Geometry check sheet. Reference: the model listing, model coordinates, mm. Face numbers are marked on the shaded views. A direction names the side the tool comes from. Coordinates: 2 decimals unless noted, no trailing zeros. Write each loop counter-clockwise with the first axis right and the second up, starting at its lowest first coordinate (ties: lowest second). Pieces come first, ordered by that corner, then holes. Notation, with made-up numbers: (78.5, 32) -> (109.5, 32) arc R13 ccw to (109.5, 50) -> close; hole circle Ø3 at (42, 12.25). An arc over 180 degrees is marked (long way). Answer in a Markdown table with one row per item. Add a question column.
Q1. Tool access check on the marked faces 4 and 5. Record the directions out of +Z, -Z, +X, -X, +Y, -Y that give a thin tool (end or side, any length) a straight path to the whole face; none if there is none.
Q2. Gauge pin test, flat ends, axial feed: P1, Ø5, axis at y = -19.5, z = 38, coming from the +X side; P2, Ø5.5, axis at x = -3.65, z = 100.03, coming from the -Y side; P3, Ø10, axis at x = 15, z = 12.5, coming from the -Y side; P4, Ø4, axis at y = -18.5, z = 45.5, coming from the +X side. Record the tip position at first contact, or that the pin passes through.
Q3. Section check A-A, the plane y = -11.5. Count the separate pieces of the cut face and the enclosed holes in it, and give its area (3 significant figures).
Q4. Section check B-B, the plane x = 31. Record the boundary of the cut face in (y, z).
Q5. Thickness scan on line 1 (Z direction, x = 0, y = -19.5) (3 decimals); line 2 (Z direction, x = 44.45, y = -17.25) (3 decimals); line 3 (Z direction, x = 1, y = -15.5). Record the ranges inside material, lowest first.
Q6. Release check for a two-part mould opening along Z. For the marked faces 1, 2 and 3 record: pulls with the +Z half, pulls with the -Z half, needs draft (parallel to the pull), parting line crosses it, or undercut.
Q7. Section check C-C, the plane z = 85.5. Record the boundary of the cut face in (x, y).
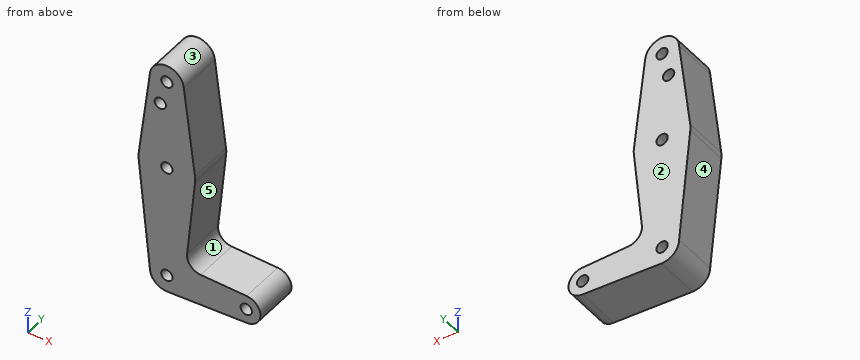
```python
from build123d import *

# Parameters (mm, degrees)
F0_R     = 3.175
F1_DEPTH = 25.4


# Not quite as in the source:
# - a feature names something its author has since deleted; it is built from what else it names


with BuildPart() as f1:
    # F0 (on Front) → F1 (new body)
    with BuildSketch(Plane.XZ):
        with BuildLine():
            ThreePointArc((-9.5149138168, 114.7382237551), (-0.2191699059, 104.7775218797), (9.525, 114.3))
            ThreePointArc((9.525, 114.3), (9.5183168712, 114.6567477241), (9.4982768633, 115.0129948306))
            ThreePointArc((9.4982768633, 115.0129948306), (-0.1376371427, 123.8240055133), (-9.5149138168, 114.7382237551))
        make_face()
        with Locations((0, 114.3)):
            Circle(F0_R, mode=Mode.SUBTRACT)
        with BuildLine():
            ThreePointArc((9.4982768633, 115.0129948306), (9.5183168712, 114.6567477241), (9.525, 114.3))
            ThreePointArc((9.525, 114.3), (-0.2191699059, 104.7775218797), (-9.5149138168, 114.7382237551))
            Line((-9.5149138168, 114.7382237551), (-15.7492887561, 65.4938727833))
            ThreePointArc((-15.7492887561, 65.4938727833), (0.002863253, 79.3749997418), (15.7500069708, 65.4881914948))
            Line((15.7500069708, 65.4881914948), (9.4982768633, 115.0129948306))
        make_face()
        with Locations((-3.6479982082, 100.0252)):
            Circle(F0_R, mode=Mode.SUBTRACT)
        with BuildLine():
            ThreePointArc((15.875, 63.5), (15.8437209276, 64.4960583162), (15.7500069708, 65.4881914948))
            ThreePointArc((15.7500069708, 65.4881914948), (0.002863253, 79.3749997418), (-15.7492887561, 65.4938727833))
            ThreePointArc((-15.7492887561, 65.4938727833), (-15.8737601653, 63.698401651), (-15.7942028036, 61.9003804205))
            ThreePointArc((-15.7942028036, 61.9003804205), (0, 47.625), (15.7942028036, 61.9003804205))
            ThreePointArc((15.7942028036, 61.9003804205), (15.8547878338, 62.6991705884), (15.875, 63.5))
        make_face()
        with Locations((0, 63.5)):
            Circle(F0_R, mode=Mode.SUBTRACT)
        with BuildLine():
            ThreePointArc((15.7942028036, 61.9003804205), (0, 47.625), (-15.7942028036, 61.9003804205))
            Line((-15.7942028036, 61.9003804205), (-9.525, 0))
            ThreePointArc((-9.525, 0), (0, 9.525), (9.525, 0))
            ThreePointArc((9.525, 0), (6.854575784, -6.6136537422), (0.3406607199, -9.5189062016))
            Line((0.3406607199, -9.5189062016), (44.5449382907, -7.9369322141))
            ThreePointArc((44.5449382907, -7.9369322141), (36.5126173213, 0.0431562547), (44.6312377373, 7.9354306205))
            Line((44.6312377373, 7.9354306205), (18.9332319933, 8.8541850706))
            ThreePointArc((18.9332319933, 8.8541850706), (13.2249062601, 11.5746494613), (11.3075490968, 17.6003984343))
            Line((11.3075490968, 17.6003984343), (15.7942028036, 61.9003804205))
        make_face()
        with BuildLine():
            ThreePointArc((9.525, 0), (0, 9.525), (-9.525, 0))
            ThreePointArc((-9.525, 0), (-6.6136537422, -6.854575784), (0.3406607199, -9.5189062016))
            ThreePointArc((0.3406607199, -9.5189062016), (6.854575784, -6.6136537422), (9.525, 0))
        make_face()
        Circle(F0_R, mode=Mode.SUBTRACT)
        with BuildLine():
            ThreePointArc((44.6312377373, 7.9354306205), (36.5126173213, 0.0431562547), (44.5449382907, -7.9369322141))
            ThreePointArc((44.5449382907, -7.9369322141), (50.0961260583, -5.5789933486), (52.3875, 0))
            ThreePointArc((52.3875, 0), (50.126375639, 5.5482128524), (44.6312377373, 7.9354306205))
        make_face()
        with Locations((44.45, 0)):
            Circle(F0_R, mode=Mode.SUBTRACT)
    extrude(amount=F1_DEPTH)


solid = f1.part
```
Calculated:
| question | item | result |
|---|---|---|
| 1 | face 4 | -Z, -X, +Y, -Y |
| 1 | face 5 | +X, +Y, -Y |
| 2 | P1 | stops at x = 13.63 |
| 2 | P2 | passes through |
| 2 | P3 | stops at y = -25.4 |
| 2 | P4 | stops at x = 14.34 |
| 3 | separate pieces | 1 |
| 3 | enclosed holes | 5 |
| 3 | area | 3,770 mm² |
| 4 | outline | (-25.4, -8.42) -> (0, -8.42) -> (0, 8.42) -> (-25.4, 8.42) -> close |
| 5 | line 1 | z = -9.525 to -3.175, 3.175 to 60.325, 66.675 to 111.125, 117.475 to 123.825 |
| 5 | line 2 | z = -7.94 to -3.175, 3.175 to 7.942 |
| 5 | line 3 | z = -9.5 to -3.01, 3.01 to 60.49, 66.51 to 111.29, 117.31 to 123.77 |
| 6 | face 1 | undercut |
| 6 | face 2 | needs draft |
| 6 | face 3 | pulls with the +Z half |
| 7 | outline | (-13.22, -25.4) -> (13.22, -25.4) -> (13.22, 0) -> (-13.22, 0) -> close |
